```python
from build123d import *

# Parameters (mm, degrees)
BOSS_EXTRU_1_DEPTH      = 4
ESQUISSE2_R             = 1.5
ENL_V_MAT_EXTRU_1_DEPTH = 4
CHANFREIN1_SIZE         = 2


with BuildPart() as part:
    # Esquisse1 → Boss.-Extru.1 (new body)
    with BuildSketch(Plane.XY):
        with BuildLine():
            Line((10, 0), (0, 0))
            Line((0, 0), (0, -26))
            ThreePointArc((0, -26), (1.464466094, -29.535533906), (5, -31))
            Line((5, -31), (55, -31))
            ThreePointArc((55, -31), (58.535533906, -29.535533906), (60, -26))
            Line((60, -26), (60, 0))
            Line((60, 0), (50, 0))
            Line((50, 0), (50, -5))
            Line((50, -5), (10, -5))
            Line((10, -5), (10, 0))
        make_face()
    extrude(amount=BOSS_EXTRU_1_DEPTH)

    # Esquisse2 → Enlèv. mat.-Extru.1 (cut)
    with BuildSketch(Plane.XY.offset(4)):
        with Locations((30, -26)):
            Circle(ESQUISSE2_R)
        with Locations((5, -5)):
            Circle(ESQUISSE2_R)
        with Locations((55, -5)):
            Circle(ESQUISSE2_R)
    extrude(amount=-ENL_V_MAT_EXTRU_1_DEPTH, mode=Mode.SUBTRACT)

    # Chanfrein1
    chanfrein1_edges = [part.edges().sort_by_distance(p)[0] for p in [
        (28.5, -26, 0),
        (3.5, -5, 0),
        (53.5, -5, 0),
    ]]
    chamfer(chanfrein1_edges, length=CHANFREIN1_SIZE)


solid = part.part
```
For this review, take the finished solid that the model builds, in its own axes (mm). A direction names the side the tool comes from. Round coordinates to 2 decimals unless told otherwise and drop trailing zeros. Write each loop counter-clockwise with the first axis right and the second up, starting at its lowest first coordinate (ties: lowest second). Pieces come first, ordered by that corner, then holes. Notation, with made-up numbers: (81, 10) - (115, 10) arc R16 cw to (115, 19) - close; hole circle Ø9 at (63.5, 48). An arc over 180 degrees is marked (long way). Put each result on its own line as item: value.
Q1. Machinability: for faces 5 (the face through (50, -2, 2)), 6 (the face through (5, 0, 2)), which of the approach directions +Z, -Z, +X, -X, +Y, -Y give a long, thin tool a straight path to every point of the face, cutting with its end or side? Answer none if there is none.
Solved:
face 5: +Z, -Z, +Y
face 6: +Z, -Z, +X, -X, +Y
Q2. We need section A-A (x = 30). Give the boundary of the cut face in (y, z), and give its area (3 significant figures).
Solved:
outline: (-31, 0) - (-29.5, 0) - (-27.5, 2) - (-27.5, 4) - (-31, 4) - close; (-24.5, 2) - (-22.5, 0) - (-5, 0) - (-5, 4) - (-24.5, 4) - close
area: 88.0 mm2
Q3. Mouldability with a two-part tool opening along X and no side actions: class faces 1 (the face through (1, -29, 2)), 2 (the face through (10, -3, 2)), 3 (the face through (30, -5, 2)), 4 (the face through (30, -31, 2)) as released by +X, released by -X, zero draft, split by the parting line, or undercut.
Solved:
face 1: released by -X
face 2: undercut
face 3: undercut
face 4: zero draft
Q4. Insertion check: pin 1 Ø3.5 at (x, y) = (55, -5) entering from -Z. The pin has a flat end and moves straight along its axis. Give the tip position at first contact, or say it passes through.
Solved:
pin 1: stops at z = 1.75
Q5. Wall thickness on probe 1 along Y at (x, z) = (30, 3.4); probe 2 along Y at (x, z) = (55, 3.5); probe 3 along Y at (x, z) = (22, 1.1): over which ranges is each line inside the solid? List them lowest first.
Solved:
probe 1: y = -31 to -27.5, -24.5 to -5
probe 2: y = -31 to -6.5, -3.5 to 0
probe 3: y = -31 to -5
Q6. We need section B-B (x = 18). Give the boundary of the cut face in (y, z), and give its area (3 significant figures).
Solved:
outline: (-31, 0) - (-5, 0) - (-5, 4) - (-31, 4) - close
area: 104 mm2
